```python
from build123d import *

# Parameters (mm, degrees)
F1_DEPTH = 5
F3_DEPTH = 25
F4_R     = 47
F5_R     = 23
F7_DEPTH = 25


with BuildPart() as f1:
    # F0 (on Front) → F1 (new body)
    with BuildSketch(Plane.XZ):
        with BuildLine():
            Line((-50, -5.5), (-50, 5.5))
            Line((-50, 5.5), (-34.9750207987, 5.5))
            ThreePointArc((-34.9750207987, 5.5), (-66, 0), (-34.9750207987, -5.5))
            Line((-34.9750207987, -5.5), (-50, -5.5))
        make_face()
        with BuildLine():
            Line((-34.9750207987, 5.5), (-50, 5.5))
            Line((-50, 5.5), (-50, -5.5))
            Line((-50, -5.5), (-34.9750207987, -5.5))
            ThreePointArc((-34.9750207987, -5.5), (-34.2456408061, -2.7928777971), (-34, 0))
            ThreePointArc((-34, 0), (-34.2456408061, 2.7928777971), (-34.9750207987, 5.5))
        make_face()
        with BuildLine():
            Line((36.044714263, 5.5), (-34.9750207987, 5.5))
            ThreePointArc((-34.9750207987, 5.5), (-34.2456408061, 2.7928777971), (-34, 0))
            ThreePointArc((-34, 0), (-34.2456408061, -2.7928777971), (-34.9750207987, -5.5))
            Line((-34.9750207987, -5.5), (36.044714263, -5.5))
            ThreePointArc((36.044714263, -5.5), (35, 0), (36.044714263, 5.5))
        make_face()
        with BuildLine():
            ThreePointArc((65, 0), (52.7991707652, 14.7365071515), (36.044714263, 5.5))
            Line((36.044714263, 5.5), (50, 5.5))
            Line((50, 5.5), (50, -5.5))
            Line((50, -5.5), (36.044714263, -5.5))
            ThreePointArc((36.044714263, -5.5), (52.7991707652, -14.7365071515), (65, 0))
        make_face()
        with BuildLine():
            Line((50, 5.5), (36.044714263, 5.5))
            ThreePointArc((36.044714263, 5.5), (35, 0), (36.044714263, -5.5))
            Line((36.044714263, -5.5), (50, -5.5))
            Line((50, -5.5), (50, 5.5))
        make_face()
    extrude(amount=F1_DEPTH)

    # F2 (on face) → F3 (cut)
    with BuildSketch(Plane.XZ.offset(5)):
        with BuildLine():
            Line((-95.8441084985, -22.139607746), (-42.6692659416, -5.8824268946))
            ThreePointArc((-42.6692659416, -5.8824268946), (-42.4482601938, 3.1912614483), (-48.2176659008, 10.1980168652))
            Line((-48.2176659008, 10.1980168652), (-100.8144274788, -5.8824268946))
            Line((-100.8144274788, -5.8824268946), (-95.8441084985, -22.139607746))
        make_face()
    extrude(amount=-F3_DEPTH, mode=Mode.SUBTRACT)

    # F4
    f4_edges = [f1.edges().sort_by_distance(p)[0] for p in [
        (-34.975021, -2.5, 5.5),
        (-34.975021, -2.5, -5.5),
    ]]
    fillet(f4_edges, radius=F4_R)

    # F5
    f5_edges = [f1.edges().sort_by_distance(p)[0] for p in [
        (36.044714, -2.5, -5.5),
        (36.044714, -2.5, 5.5),
    ]]
    fillet(f5_edges, radius=F5_R)

    # F6 (on face) → F7 (cut)
    with BuildSketch(Plane.XZ.offset(5)):
        with BuildLine():
            Line((72.8835861022, 14.825997855), (47.0633576912, 6.9319618275))
            ThreePointArc((47.0633576912, 6.9319618275), (46.3099800667, -0.0953652442), (50.8641898526, -5.5))
            Line((50.8641898526, -5.5), (76.6844182636, 2.3940360275))
            Line((76.6844182636, 2.3940360275), (72.8835861022, 14.825997855))
        make_face()
    extrude(amount=-F7_DEPTH, mode=Mode.SUBTRACT)


solid = f1.part
```
Here's how the part is built. I have some questions about the finished solid (model axes, mm). A direction names the side the tool comes from. Coordinates: 2 decimals unless noted, no trailing zeros. Order: outer loops, then holes, each group sorted by start corner. A loop starts at its lowest first (then second) coordinate and runs counter-clockwise, first axis right, second up.
1) We'd pull the mould along X, two halves only. Please class faces 4 (the face through (53.744, -2.535, 8.974)), 5 (the face through (5, -2, -5.5)), 6 (the face through (-1, 0, 0)): +X half, -X half, draft (parallel to the pull), parting line (faces both ways), or undercut.
2) Which directions (+Z, -Z, +X, -X, +Y, -Y) give clear straight access to the entire face, cutting with the end or side of a thin tool? Please do faces 1 (the face through (-52.02, -2.54, -8.74)), 2 (the face through (5, -2, 5.5)), 3 (the face through (-28.559, -2.535, -7.446)).
3) Imagine slicing it at B-B on z = -7.5. List the corners of the cut face in (x, y) for me.
4) Will these pins go through, and if not, where does the flat tip stop? pin 1 (2 mm diameter, centred on x = -4, z = -7.5, fed in from -Y); pin 2 (1.5 mm diameter, centred on x = 13.5, y = -1.5, fed in from -Z); pin 3 (1.5 mm diameter, centred on x = 37.5, y = -4, fed in from +Z).
5) I need wall thicknesses on line 1 (Z direction, x = 57, y = -4.8); line 2 (X direction, y = -0.85, z = -13); line 3 (Z direction, x = 13.5, y = -1.2). Which ranges of each line are inside material? Lowest first, please.
6) Imagine slicing it at C-C on x = -11.5. List the corners of the cut face in (y, z) for me.
7) Imagine slicing it at A-A on y = -2.15. List the corners of the cut face in (x, z) for me, and give its area (3 significant figures).
8) Imagine slicing it at D-D on x = -32.5. List the corners of the cut face in (y, z) for me, and give its area (3 significant figures).
Response values:
1. face 4: +X half
1. face 5: undercut
1. face 6: draft
2. face 1: -X, +Y, -Y
2. face 2: +Z, +Y, -Y
2. face 3: -Z, +Y, -Y
3. outline: (-47.96, -5) - (-28.74, -5) - (-28.74, 0) - (-47.96, 0) - close; (34.25, -5) - (62.99, -5) - (62.99, 0) - (34.25, 0) - close
4. pin 1: passes through
4. pin 2: stops at z = -5.5
4. pin 3: stops at z = 9.8
5. line 1: z = -13.27 to -3.62, 9.97 to 13.27
5. line 2: x = -59.33 to -40.65, 42.52 to 57.48
5. line 3: z = -5.5 to 5.5
6. outline: (-5, -5.5) - (0, -5.5) - (0, 5.5) - (-5, 5.5) - close
7. outline: (-65.2, 5.01) - (-48.22, 10.2) arc R13 cw to (-42.67, -5.88) - (-61.1, -11.52) arc R16 ccw to (-41.16, -13.33) arc R47 cw to (-15.18, -5.5) - (24.87, -5.5) arc R23 cw to (40.08, -11.25) arc R15 ccw to (64.95, -1.19) - (50.86, -5.5) arc R9 cw to (47.06, 6.93) - (60.24, 10.96) arc R15 ccw to (40.08, 11.25) arc R23 cw to (24.87, 5.5) - (-15.18, 5.5) arc R47 cw to (-41.16, 13.33) arc R16 ccw to start
7. area: 1,770 mm2
8. outline: (-5, -8.81) - (0, -8.81) - (0, 8.81) - (-5, 8.81) - close
8. area: 88.1 mm2
